Can you work these out from the model? Positions are in its coordinate system, mm. Face numbers are marked on the shaded views. A direction names the side the tool comes from. Give positions to 0.01 mm unless a question says otherwise; leave off trailing zeros. Order: outer loops, then holes, each group sorted by start corner. A loop starts at its lowest first (then second) coordinate and runs counter-clockwise, first axis right, second up.
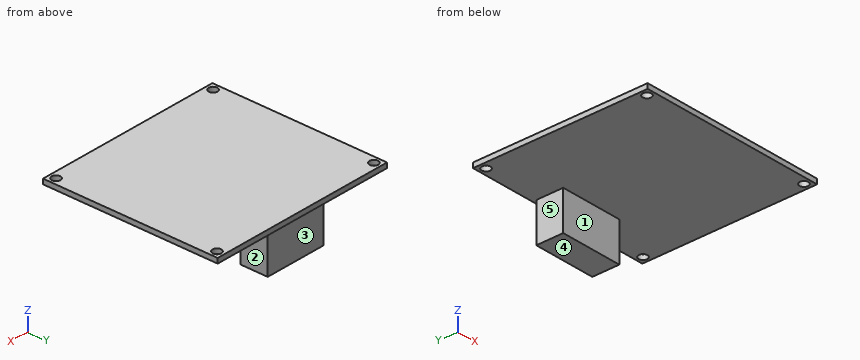
```python
from build123d import *

# Parameters (mm, degrees)
SKETCH1_W           = 63.119
SKETCH1_H           = 58.42
BOSS_EXTRUDE1_DEPTH = 0.8255
SKETCH6_W           = 20.8788
SKETCH6_H           = 9.017
BOSS_EXTRUDE3_DEPTH = 13.081
SKETCH3_R           = 1.4605
CUT_EXTRUDE1_DEPTH  = 15.732


with BuildPart() as part:
    # Sketch1 → Boss-Extrude1 (new body, symmetric)
    with BuildSketch(Plane.XY):
        Rectangle(SKETCH1_W, SKETCH1_H)
    extrude(amount=BOSS_EXTRUDE1_DEPTH, both=True)

    # Sketch6 → Boss-Extrude3 (add)
    with BuildSketch(Plane(origin=(0, 0, -0.8255), x_dir=(-1, 0, 0), z_dir=(0, 0, -1))):
        with Locations((-1.0541, 23.4315)):
            Rectangle(SKETCH6_W, SKETCH6_H)
    extrude(amount=BOSS_EXTRUDE3_DEPTH)

    # Sketch3 → Cut-Extrude1 (cut, through all)
    with BuildSketch(Plane.XY.offset(0.8255)):
        with Locations((-29.25826, 26.9113)):
            Circle(SKETCH3_R)
        with Locations((29.25826, 26.9113)):
            Circle(SKETCH3_R)
        with Locations((29.25826, -26.9113)):
            Circle(SKETCH3_R)
        with Locations((-29.25826, -26.9113)):
            Circle(SKETCH3_R)
    extrude(amount=-CUT_EXTRUDE1_DEPTH, mode=Mode.SUBTRACT)


solid = part.part
```
1) Which directions (+Z, -Z, +X, -X, +Y, -Y) give clear straight access to the entire face, cutting with the end or side of a thin tool? Please do the marked faces 1, 2, 3, 4 and 5.
2) Suppose I cut it at A-A (x = 7). Please give me the cut outline in (y, z).
3) I'm going to push flat-ended pins straight in: pin 1 Ø3.5 at (x, y) = (29.26, 26.91) entering from +Z; pin 2 Ø12 at (x, y) = (2, -6) entering from -Z; pin 3 Ø1.5 at (y, z) = (22.5, -11.5) entering from -X; pin 4 Ø4.5 at (y, z) = (21.5, -4.5) entering from +X. Where does each tip first touch, or does it pass through?
4) Suppose I cut it at B-B (z = -3). Please give me the cut outline in (x, y), and give its area (3 significant figures).
5) If I drill on line 1 (X direction, y = 26, z = -2.75); line 2 (Z direction, x = 4.5, y = -26); line 3 (Y direction, x = 4.5, z = -4), over which ranges is the centre line in solid material (lowest first)?
6) Suppose I cut it at C-C (y = -16). Please give me the cut outline in (x, z).
Results:
1. face 1: -Z, +X, -X, -Y
1. face 2: -Z, +X, +Y, -Y
1. face 3: -Z, +X, -X, +Y
1. face 4: -Z, +X, -X, +Y, -Y
1. face 5: -Z, -X, +Y, -Y
2. outline: (-29.21, -0.83) - (18.92, -0.83) - (18.92, -13.91) - (27.94, -13.91) - (27.94, -0.83) - (29.21, -0.83) - (29.21, 0.83) - (-29.21, 0.83) - close
3. pin 1: stops at z = 0.83
3. pin 2: stops at z = -0.83
3. pin 3: stops at x = -9.39
3. pin 4: stops at x = 11.49
4. outline: (-9.39, 18.92) - (11.49, 18.92) - (11.49, 27.94) - (-9.39, 27.94) - close
4. area: 188 mm2
5. line 1: x = -9.39 to 11.49
5. line 2: z = -0.83 to 0.83
5. line 3: y = 18.92 to 27.94
6. outline: (-31.56, -0.83) - (31.56, -0.83) - (31.56, 0.83) - (-31.56, 0.83) - close
